The listing builds one solid part. Answer for the finished solid, in the listing's coordinates (mm). Face numbers are marked on the shaded views. A direction names the side the tool comes from. Coordinates: 2 decimals unless noted, no trailing zeros. Loops run counter-clockwise (first coordinate to the right, second up) from the corner with the lowest first, then second, coordinate; pieces in that order, holes last. Notation, with made-up numbers: M 76,2 L 106,2 A16 cw 106,29 Z; hole C 78,29 d8. An arc over 180 degrees is marked long. Answer in a Markdown table with one row per item. Add a question column.
from build123d import *

# Parameters (mm, degrees)
SKETCH1_W               = 33.25
SKETCH1_H               = 12
BOSS_EXTRUDE1_DEPTH     = 3.25
CUT_EXTRUDE1_DEPTH      = 36.498239393
CUT_EXTRUDE1_DEPTH_BACK = 36.498239393
SKETCH2_R               = 2.2
SKETCH3_W               = 3.25
SKETCH3_H               = 12
BOSS_EXTRUDE2_DEPTH     = 30
SKETCH4_R               = 2.2
CUT_EXTRUDE2_DEPTH      = 47.363374554
FILLET2_R               = 5.75
FILLET3_R               = 2.5


with BuildPart() as part:
    # Sketch1 → Boss-Extrude1 (new body)
    with BuildSketch(Plane(origin=(0, 0, 0), x_dir=(1, 0, 0), z_dir=(0, 1, 0))):
        with Locations((-16.625, 6)):
            Rectangle(SKETCH1_W, SKETCH1_H)
    extrude(amount=BOSS_EXTRUDE1_DEPTH)

    # Sketch2 → Cut-Extrude1 (cut, two sides: drawn at the far end of the back side and taken through both)
    with BuildSketch(Plane(origin=(0, 3.25, 0), x_dir=(1, 0, 0), z_dir=(0, 1, 0)).offset(-CUT_EXTRUDE1_DEPTH_BACK)):
        with Locations(Location((-27.25, 6, 0), (0, 0, 270))):
            Circle(SKETCH2_R)
    extrude(amount=CUT_EXTRUDE1_DEPTH + CUT_EXTRUDE1_DEPTH_BACK, mode=Mode.SUBTRACT)

    # Sketch3 → Boss-Extrude2 (add)
    with BuildSketch(Plane.XZ):
        with Locations((-1.625, -6)):
            Rectangle(SKETCH3_W, SKETCH3_H)
    extrude(amount=BOSS_EXTRUDE2_DEPTH)

    # Sketch4 → Cut-Extrude2 (cut, through all)
    with BuildSketch(Plane(origin=(0, 0, 0), x_dir=(0, 0, -1), z_dir=(1, 0, 0))):
        with Locations((6, -24)):
            Circle(SKETCH4_R)
    extrude(amount=-CUT_EXTRUDE2_DEPTH, mode=Mode.SUBTRACT)

    # Fillet2
    fillet2_edges = [part.edges().sort_by_distance(p)[0] for p in [
        (0, 3.25, -6),
    ]]
    fillet(fillet2_edges, radius=FILLET2_R)

    # Fillet3
    fillet3_edges = [part.edges().sort_by_distance(p)[0] for p in [
        (-3.25, 0, -6),
    ]]
    fillet(fillet3_edges, radius=FILLET3_R)


solid = part.part
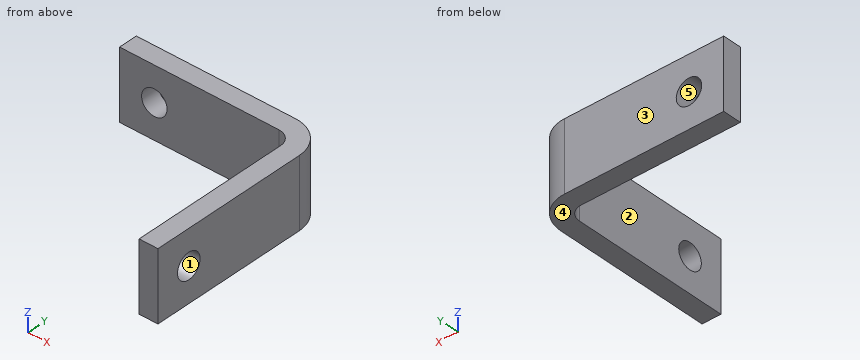
(1) For the marked faces 1 and 2, determine the directions among +Z, -Z, +X, -X, +Y, -Y from which every point of the face is accessible in a straight line to the end or side of a thin tool.
(2) A cutting plane is placed at A-A (x = -27.25). Give the vertices of the cut face in (y, z).
(3) A cutting plane is placed at B-B (z = -5.25). Give the vertices of the cut face in (x, y).
(4) A cutting plane is placed at D-D (x = -22). Give the vertices of the cut face in (y, z), plus the area to 3 significant figures.
(5) Straight lines are drawn through the part: line 1 (Z direction, x = -27.25, y = 2.15); line 2 (Y direction, x = -12, z = -2.5). For each, find the intervals that lie inside material, in ascending order.
(6) The mould has two halves that part along Z. Classify the marked faces 3, 4 and 5: released by +Z, released by -Z, zero draft, split by the parting line, or undercut.
(7) Each of these flat-tipped pins is pushed along its axis until it touches: pin 1 (3 mm diameter, centred on x = -25.5, z = -4, fed in from -Y); pin 2 (4 mm diameter, centred on x = -27.25, z = -6, fed in from -Y); pin 3 (5 mm diameter, centred on y = -17.5, z = -2, fed in from -X); pin 4 (5.5 mm diameter, centred on y = -24, z = -6, fed in from +X). Where does it stop, or does it pass through?
(8) A cutting plane is placed at C-C (z = -2.25). Give the vertices of the cut face in (x, y), plus the area to 3 significant figures.
Solved:
| question | item | result |
|---|---|---|
| 1 | face 1 | +X, -X |
| 1 | face 2 | +Z, -Z, -X, -Y |
| 2 | outline | M 0,-12 L 3.25,-12 L 3.25,-8.2 L 0,-8.2 Z; M 0,-3.8 L 3.25,-3.8 L 3.25,0 L 0,0 Z |
| 3 | outline | M -33.25,0 L -29.32,0 L -29.32,3.25 L -33.25,3.25 Z; M -25.18,0 L -5.75,0 A2.5 cw -3.25,-2.5 L -3.25,-21.93 L 0,-21.93 L 0,-2.5 A5.75 ccw -5.75,3.25 L -25.18,3.25 Z; M -3.25,-30 L 0,-30 L 0,-26.07 L -3.25,-26.07 Z |
| 4 | outline | M 0,-12 L 3.25,-12 L 3.25,0 L 0,0 Z |
| 4 | area | 39.0 mm² |
| 5 | line 1 | z = -12 to -8.2, -3.8 to 0 |
| 5 | line 2 | y = 0 to 3.25 |
| 6 | face 3 | zero draft |
| 6 | face 4 | released by -Z |
| 6 | face 5 | undercut |
| 7 | pin 1 | stops at y = 0 |
| 7 | pin 2 | passes through |
| 7 | pin 3 | stops at x = -3.25 |
| 7 | pin 4 | stops at x = 0 |
| 8 | outline | M -33.25,0 L -5.75,0 A2.5 cw -3.25,-2.5 L -3.25,-30 L 0,-30 L 0,-2.5 A5.75 ccw -5.75,3.25 L -33.25,3.25 Z |
| 8 | area | 200 mm² |
